Can you work these out from the model? Positions are in its coordinate system, mm. A direction names the side the tool comes from. Round coordinates to 2 decimals unless told otherwise and drop trailing zeros. Write each loop counter-clockwise with the first axis right and the second up, starting at its lowest first coordinate (ties: lowest second). Pieces come first, ordered by that corner, then holes.
Q1. I'm going to push a flat-ended pin straight in: pin 1 Ø12 at (x, z) = (-29.5, 14.5) entering from -Y. Where does the tip first touch, or does it pass through?
Q2. If we section it at C-C (z = -35.5): Please give me the cut outline in (x, y).
Q3. If we section it at B-B (y = 2.25): Please give me the cut outline in (x, z).
Q4. For faces 1 (the flat face through (-1, 3, -42.5)), 2 (the flat face through (33, 21, -47)), which set-ups out of +Z, -Z, +X, -X, +Y, -Y let a thin tool reach every point of the face, with its end or its side?
Q5. If we section it at D-D (y = 7.75): Please give me the cut outline in (x, z).
Q6. We'd pull the mould along Z, two halves only. Please class faces 3 (the flat face through (1, 10, 47.5)), 4 (the flat face through (47.5, 10, -1)), 5 (the flat face through (-1, 3, 42.5)): +Z half, -Z half, draft (parallel to the pull), parting line (faces both ways), or undercut.
Q7. If we section it at A-A (x = -13.5): Please give me the cut outline in (y, z).
Q8. Please list where these lines run through material, in increasing order: line 1 along Z through (x, y) = (-37, 2.75); line 2 along X through (y, z) = (14, 23.5).
from build123d import *

# Parameters (mm, degrees)
BOSS_EXTRUDE1_DEPTH = 4
SKETCH4_W           = 91
SKETCH4_H           = 91
BOSS_EXTRUDE2_DEPTH = 15
CUT_EXTRUDE3_REACH  = 70.829
SKETCH2_W           = 80
SKETCH2_H           = 80
CUT_EXTRUDE6_REACH  = 109.899
SKETCH7_W           = 10
SKETCH7_H           = 1
SKETCH8_W           = 85
SKETCH8_H           = 85
CUT_EXTRUDE7_DEPTH  = 3
BOSS_EXTRUDE3_DEPTH = 2
CHAMFER1_SIZE       = 0.5
CUT_EXTRUDE8_REACH  = 110.269
SKETCH11_W          = 9.5
SKETCH11_H          = 1
CUT_EXTRUDE10_DEPTH = 1


with BuildPart() as part:
    # Sketch1 → Boss-Extrude1 (new body)
    with BuildSketch(Plane(origin=(0, 0, 0), x_dir=(1, 0, 0), z_dir=(0, 1, 0))):
        with BuildLine():
            Line((-46.5, -47.5), (46.5, -47.5))
            ThreePointArc((46.5, -47.5), (47.207106781, -47.207106781), (47.5, -46.5))
            Line((47.5, -46.5), (47.5, 46.5))
            ThreePointArc((47.5, 46.5), (47.207106781, 47.207106781), (46.5, 47.5))
            Line((46.5, 47.5), (-46.5, 47.5))
            ThreePointArc((-46.5, 47.5), (-47.207106781, 47.207106781), (-47.5, 46.5))
            Line((-47.5, 46.5), (-47.5, -46.5))
            ThreePointArc((-47.5, -46.5), (-47.207106781, -47.207106781), (-46.5, -47.5))
        make_face()
    extrude(amount=BOSS_EXTRUDE1_DEPTH)

    # Sketch4 → Boss-Extrude2 (add)
    with BuildSketch(Plane(origin=(0, 4, 0), x_dir=(1, 0, 0), z_dir=(0, 1, 0))):
        with BuildLine():
            Line((47.5, -46.5), (47.5, 46.5))
            ThreePointArc((47.5, 46.5), (47.207106781, 47.207106781), (46.5, 47.5))
            Line((46.5, 47.5), (-46.5, 47.5))
            ThreePointArc((-46.5, 47.5), (-47.207106781, 47.207106781), (-47.5, 46.5))
            Line((-47.5, 46.5), (-47.5, -46.5))
            ThreePointArc((-47.5, -46.5), (-47.207106781, -47.207106781), (-46.5, -47.5))
            Line((-46.5, -47.5), (46.5, -47.5))
            ThreePointArc((46.5, -47.5), (47.207106781, -47.207106781), (47.5, -46.5))
        make_face()
        Rectangle(SKETCH4_W, SKETCH4_H, mode=Mode.SUBTRACT)
    extrude(amount=BOSS_EXTRUDE2_DEPTH)

    # Sketch2 → Cut-Extrude3 (cut, up to next)
    with BuildSketch(Plane(origin=(0, 4, 0), x_dir=(1, 0, 0), z_dir=(0, 1, 0)), mode=Mode.PRIVATE) as cut_extrude3_sk1:
        Rectangle(SKETCH2_W, SKETCH2_H)
    cut_extrude3_tool1 = extrude(cut_extrude3_sk1.sketch, amount=-CUT_EXTRUDE3_REACH, mode=Mode.PRIVATE) & part.part
    add(cut_extrude3_tool1.solids().sort_by_distance((0, 4, 0))[0], mode=Mode.SUBTRACT)

    # Sketch7 → Cut-Extrude6 (cut, up to next)
    with BuildSketch(Plane(origin=(47.5, 0, 0), x_dir=(0, 0, -1), z_dir=(1, 0, 0)), mode=Mode.PRIVATE) as cut_extrude6_sk1:
        with Locations((0, 18.5)):
            Rectangle(SKETCH7_W, SKETCH7_H)
    cut_extrude6_tool1 = extrude(cut_extrude6_sk1.sketch, amount=-CUT_EXTRUDE6_REACH, mode=Mode.PRIVATE) & part.part
    add(cut_extrude6_tool1.solids().sort_by_distance((47.5, 18.5, 0))[0], mode=Mode.SUBTRACT)

    # Sketch8 → Cut-Extrude7 (cut)
    with BuildSketch(Plane(origin=(0, 4, 0), x_dir=(1, 0, 0), z_dir=(0, 1, 0))):
        Rectangle(SKETCH8_W, SKETCH8_H)
    extrude(amount=-CUT_EXTRUDE7_DEPTH, mode=Mode.SUBTRACT)

    # Sketch10 → Boss-Extrude3 (add)
    with BuildSketch(Plane(origin=(0, 19, 0), x_dir=(1, 0, 0), z_dir=(0, 1, 0))):
        with BuildLine():
            Line((46.5, 5), (46.5, 46.5))
            Line((46.5, 46.5), (-46.5, 46.5))
            Line((-46.5, 46.5), (-46.5, -46.5))
            Line((-46.5, -46.5), (46.5, -46.5))
            Line((46.5, -46.5), (46.5, -5))
            Line((46.5, -5), (47.5, -5))
            Line((47.5, -5), (47.5, -46.5))
            ThreePointArc((47.5, -46.5), (47.207106781, -47.207106781), (46.5, -47.5))
            Line((46.5, -47.5), (-46.5, -47.5))
            ThreePointArc((-46.5, -47.5), (-47.207106781, -47.207106781), (-47.5, -46.5))
            Line((-47.5, -46.5), (-47.5, 46.5))
            ThreePointArc((-47.5, 46.5), (-47.207106781, 47.207106781), (-46.5, 47.5))
            Line((-46.5, 47.5), (46.5, 47.5))
            ThreePointArc((46.5, 47.5), (47.207106781, 47.207106781), (47.5, 46.5))
            Line((47.5, 46.5), (47.5, 5))
            Line((47.5, 5), (46.5, 5))
        make_face()
    extrude(amount=BOSS_EXTRUDE3_DEPTH)

    # Chamfer1
    chamfer1_edges = [part.edges().sort_by_distance(p)[0] for p in [
        (47, 21, 5),
        (47, 21, -5),
        (45.5, 18.5, -5),
        (45.5, 18, 0),
        (46.5, 18, -5),
        (46, 19, 5),
    ]]
    chamfer(chamfer1_edges, length=CHAMFER1_SIZE)

    # Sketch11 → Cut-Extrude8 (cut, up to next)
    with BuildSketch(Plane(origin=(0, 0, -47.5), x_dir=(-1, 0, 0), z_dir=(0, 0, -1)), mode=Mode.PRIVATE) as cut_extrude8_sk1:
        with Locations((11.25, 20.5)):
            Rectangle(SKETCH11_W, SKETCH11_H)
    cut_extrude8_tool1 = extrude(cut_extrude8_sk1.sketch, amount=-CUT_EXTRUDE8_REACH, mode=Mode.PRIVATE) & part.part
    add(cut_extrude8_tool1.solids().sort_by_distance((-11.25, 20.5, -47.5))[0], mode=Mode.SUBTRACT)

    # Sketch12 → Cut-Extrude10 (cut)
    with BuildSketch(Plane(origin=(0, 0, -47.5), x_dir=(-1, 0, 0), z_dir=(0, 0, -1))):
        Polygon((16, 20), (16, 21), (18, 21), (18, 18), (4.5, 18), (4.5, 21), (6.5, 21), (6.5, 20), align=None)
    extrude(amount=-CUT_EXTRUDE10_DEPTH, mode=Mode.SUBTRACT)


solid = part.part
A:
1. pin 1: passes through
2. outline: (-47.5, 0) - (-40, 0) - (-40, 1) - (-42.5, 1) - (-42.5, 4) - (-45.5, 4) - (-45.5, 19) - (-46.5, 19) - (-46.5, 21) - (-47.5, 21) - close; (40, 0) - (47.5, 0) - (47.5, 21) - (46.5, 21) - (46.5, 19) - (45.5, 19) - (45.5, 4) - (42.5, 4) - (42.5, 1) - (40, 1) - close
3. outline: (-47.5, -46.5) arc R1 ccw to (-46.5, -47.5) - (46.5, -47.5) arc R1 ccw to (47.5, -46.5) - (47.5, 46.5) arc R1 ccw to (46.5, 47.5) - (-46.5, 47.5) arc R1 ccw to (-47.5, 46.5) - close; hole (-42.5, -42.5) - (42.5, -42.5) - (42.5, 42.5) - (-42.5, 42.5) - close
4. face 1: +Y
4. face 2: +Z, -Z, +X, -X, +Y
5. outline: (-47.5, -46.5) arc R1 ccw to (-46.5, -47.5) - (46.5, -47.5) arc R1 ccw to (47.5, -46.5) - (47.5, 46.5) arc R1 ccw to (46.5, 47.5) - (-46.5, 47.5) arc R1 ccw to (-47.5, 46.5) - close; hole (-45.5, -45.5) - (45.5, -45.5) - (45.5, 45.5) - (-45.5, 45.5) - close
6. face 3: +Z half
6. face 4: draft
6. face 5: undercut
7. outline: (0, -47.5) - (18, -47.5) - (18, -46.5) - (19, -46.5) - (19, -45.5) - (4, -45.5) - (4, -42.5) - (1, -42.5) - (1, -40) - (0, -40) - close; (0, 40) - (1, 40) - (1, 42.5) - (4, 42.5) - (4, 45.5) - (19, 45.5) - (19, 46.5) - (21, 46.5) - (21, 47.5) - (0, 47.5) - close
8. line 1: z = -47.5 to -42.5, 42.5 to 47.5
8. line 2: x = -47.5 to -45.5, 45.5 to 47.5
